The listing builds one solid part. Answer for the finished solid, in the listing's coordinates (mm). A direction names the side the tool comes from. Coordinates: 2 decimals unless noted, no trailing zeros. Order: outer loops, then holes, each group sorted by start corner. A loop starts at its lowest first (then second) coordinate and runs counter-clockwise, first axis right, second up. Notation, with made-up numbers: (42.25, 12) -> (49.25, 12) arc R20 cw to (49.25, 17) -> close; hole circle Ø8 at (70.25, -25). An arc over 180 degrees is marked (long way). Answer in a Markdown table with one row per item.
```python
from build123d import *

# Parameters (mm, degrees)
SKETCH2_R           = 2.778125
EXTRUDE1_DEPTH      = 19.05
EXTRUDE1_DEPTH_BACK = 19.05
CHAMFER1_SIZE       = 0.555625
CUT_EXTRUDE1_DEPTH  = 7.62
SKETCH5_R           = 1.190625
CUT_EXTRUDE2_DEPTH  = 5.02828125


with BuildPart() as part:
    # Sketch2 → Extrude1 (new body, two sides)
    with BuildSketch(Plane(origin=(0, 0, 0), x_dir=(0, 0, -1), z_dir=(1, 0, 0))) as extrude1_sk:
        Circle(SKETCH2_R)
    extrude(amount=EXTRUDE1_DEPTH)
    extrude(extrude1_sk.sketch, amount=-EXTRUDE1_DEPTH_BACK)

    # Chamfer1
    chamfer1_edges = [part.edges().sort_by_distance(p)[0] for p in [
        (-19.05, 0, 2.778125),
        (19.05, 0, 2.778125),
    ]]
    chamfer(chamfer1_edges, length=CHAMFER1_SIZE)

    # Sketch3 → Cut-Extrude1 (cut)
    with BuildSketch(Plane.ZY.offset(19.05)):
        with BuildLine():
            Line((-3.175, 3.175), (-3.175, -3.175))
            Line((-3.175, -3.175), (-1.25015625, -3.175))
            Line((-1.25015625, -3.175), (-1.25015625, -1.837556965))
            ThreePointArc((-1.25015625, -1.837556965), (-2.2225, 0), (-1.25015625, 1.837556965))
            Line((-1.25015625, 1.837556965), (-1.25015625, 3.175))
            Line((-1.25015625, 3.175), (-3.175, 3.175))
        make_face()
        with BuildLine():
            Line((1.25015625, -1.837556965), (1.25015625, -3.175))
            Line((1.25015625, -3.175), (3.175, -3.175))
            Line((3.175, -3.175), (3.175, 3.175))
            Line((3.175, 3.175), (1.25015625, 3.175))
            Line((1.25015625, 3.175), (1.25015625, 1.837556965))
            ThreePointArc((1.25015625, 1.837556965), (1.964431026, 1.039479193), (2.2225, 0))
            ThreePointArc((2.2225, 0), (1.964431026, -1.039479193), (1.25015625, -1.837556965))
        make_face()
        with BuildLine():
            ThreePointArc((-1.25015625, 1.837556965), (-2.2225, 0), (-1.25015625, -1.837556965))
            Line((-1.25015625, -1.837556965), (-1.25015625, 1.837556965))
        make_face()
        with BuildLine():
            Line((1.25015625, 1.837556965), (1.25015625, -1.837556965))
            ThreePointArc((1.25015625, -1.837556965), (1.964431026, -1.039479193), (2.2225, 0))
            ThreePointArc((2.2225, 0), (1.964431026, 1.039479193), (1.25015625, 1.837556965))
        make_face()
    extrude(amount=-CUT_EXTRUDE1_DEPTH, mode=Mode.SUBTRACT)

    # Sketch5 → Cut-Extrude2 (cut, through all)
    with BuildSketch(Plane.XY.offset(1.25015625)):
        with Locations((-15.24, 0)):
            Circle(SKETCH5_R)
    extrude(amount=-CUT_EXTRUDE2_DEPTH, mode=Mode.SUBTRACT)


solid = part.part
```
(1) A cutting plane is placed at B-B, the plane y = 0. Determine the outline of the cut face in (x, z), then the cut area to 3 significant figures.
Check values:
| item | result |
|---|---|
| outline | (-19.05, -1.25) -> (-16.43, -1.25) -> (-16.43, 1.25) -> (-19.05, 1.25) -> close; (-14.05, -1.25) -> (-11.43, -1.25) -> (-11.43, -2.78) -> (18.49, -2.78) -> (19.05, -2.22) -> (19.05, 2.22) -> (18.49, 2.78) -> (-11.43, 2.78) -> (-11.43, 1.25) -> (-14.05, 1.25) -> close |
| area | 182 mm² |
(2) Find the intervals of material crossed by line 1 along Y through (x, z) = (-15.24, 0); line 2 along X through (y, z) = (-0.25, -1.95); line 3 along Y through (x, z) = (-15.24, -0.5), in increasing order. Write a range as from..to.
Check values:
| item | result |
|---|---|
| line 1 | -2.78..-1.19, 1.19..2.78 |
| line 2 | -11.43..19.05 |
| line 3 | -2.73..-1.19, 1.19..2.73 |
(3) A cutting plane is placed at C-C, the plane x = -15.24. Determine the outline of the cut face in (y, z).
Check values:
| item | result |
|---|---|
| outline | (-2.48, -1.25) -> (-1.19, -1.25) -> (-1.19, 1.25) -> (-2.48, 1.25) arc R2.78 ccw to start; (1.19, -1.25) -> (2.48, -1.25) arc R2.78 ccw to (2.48, 1.25) -> (1.19, 1.25) -> close |
(4) Which of the six approach directions +Z, -Z, +X, -X, +Y, -Y give full straight-line access (tool end or side, diameter ignored) to faces 1 (the flat face through (-11.43, 0, 2)), 2 (the flat face through (-11.43, 0, -2)), 3 (the flat face through (-19.05, 0, 0))?
Check values:
| item | result |
|---|---|
| face 1 | +Z, -X, +Y, -Y |
| face 2 | -Z, -X, +Y, -Y |
| face 3 | +Z, -Z, -X, +Y, -Y |
(5) A cutting plane is placed at D-D, the plane x = -1. Determine the outline of the cut face in (y, z).
Check values:
| item | result |
|---|---|
| outline | circle Ø5.56 at (0, 0) |
(6) For a pull along X with two mould halves and no side action, classify faces 4 (the cylindrical face through (4.369, 0.122, 2.775)), 5 (the flat face through (19.05, 0, 0)), 6 (the conical face through (-18.84, 2.43, -0.02)), 7 (the cylindrical face through (-14.104, 0.358, 0.018)) as released by +X, released by -X, zero draft, split by the parting line, or undercut.
Check values:
| item | result |
|---|---|
| face 4 | zero draft |
| face 5 | released by +X |
| face 6 | released by -X |
| face 7 | undercut |
(7) A cutting plane is placed at A-A, the plane z = 0. Determine the outline of the cut face in (x, y), then the cut area to 3 significant figures.
Check values:
| item | result |
|---|---|
| outline | (-19.05, -2.22) -> (-18.49, -2.78) -> (18.49, -2.78) -> (19.05, -2.22) -> (19.05, 2.22) -> (18.49, 2.78) -> (-18.49, 2.78) -> (-19.05, 2.22) -> close; hole circle Ø2.38 at (-15.24, 0) |
| area | 207 mm² |
(8) Flat-ended cylindrical pins translate along their axes: pin 1 (1.5 mm diameter, centred on x = 10.5, y = 0.5, fed in from +Z); pin 2 (0.8 mm diameter, centred on y = -0.5, z = 2.5, fed in from -X). Find the tip coordinate at first contact, or state that the pin passes through.
Check values:
| item | result |
|---|---|
| pin 1 | z = 2.78 |
| pin 2 | x = -11.43 |
